The figure shows three views and two pictorial views of one solid part (mm, origin at its lowest corner). Answer the questions. A direction names the side the tool comes from. Coordinates: 2 decimals unless noted, no trailing zeros. Loops run counter-clockwise (first coordinate to the right, second up) from the corner with the lowest first, then second, coordinate; pieces in that order, holes last. Notation, with made-up numbers: (78, 22.5) -> (110, 22.5) arc R33 ccw to (110, 54.5) -> close; hole circle Ø10 at (43.25, -18.75). An arc over 180 degrees is marked (long way). Answer as a JSON object with one key per item and string values. Group by question number.
1) Consider probe 1 along X at (y, z) = (17.5, 16); probe 2 along Y at (x, z) = (56, 30). Determine where each line is inside the solid, lowest interval first. Write a range as [from, to].
2) Section C-C, the plane y = 18.75 is taken. Give the vertices of the cut face in (x, z).
3) Section B-B, the plane z = 30 is taken. Give the vertices of the cut face in (x, y).
4) Which of the six approach directions +Z, -Z, +X, -X, +Y, -Y give full straight-line access (tool end or side, diameter ignored) to the marked faces 1 and 2?
5) Section D-D, the plane z = 44.5 is taken. Give the vertices of the cut face in (x, y), plus the area to 3 significant figures.
6) Section A-A, the plane y = 12.5 is taken. Give the vertices of the cut face in (x, z).
7) Flat-ended cylindrical pins translate along their axes: P1, Ø4, axis at y = 12.5, z = 30, coming from the +X side; P2, Ø1.5, axis at x = 13, z = 33, coming from the +Y side. Find the tip coordinate at first contact, or state that the pin passes through.
8) Determine the mould class of the marked faces 3, 4, 5 and 6 for opening direction Z: released by +Z, released by -Z, zero draft, split by the parting line, or undercut.
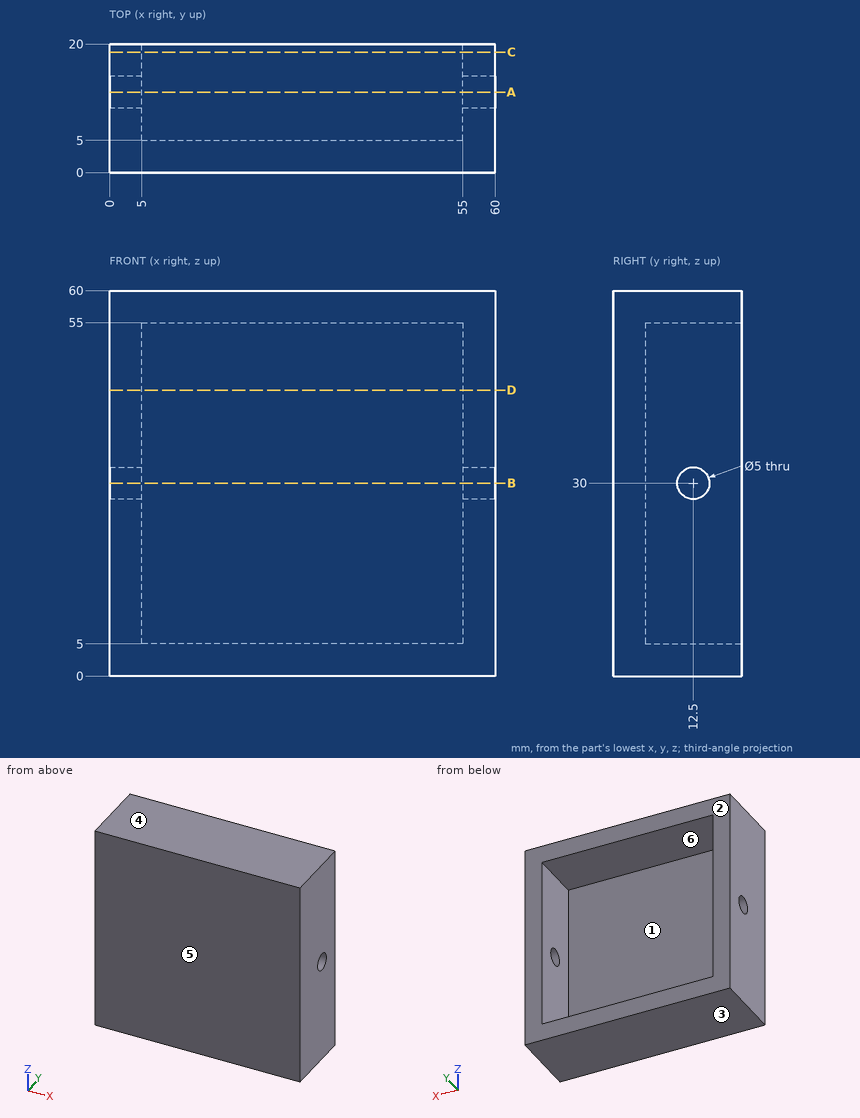
Determined:
{
 "1": {"probe 1": "[0, 5], [55, 60]", "probe 2": "[0, 10], [15, 20]"},
 "2": {"outline": "(0, 0) -> (60, 0) -> (60, 60) -> (0, 60) -> close; hole (5, 5) -> (55, 5) -> (55, 55) -> (5, 55) -> close"},
 "3": {"outline": "(0, 0) -> (60, 0) -> (60, 10) -> (55, 10) -> (55, 5) -> (5, 5) -> (5, 10) -> (0, 10) -> close; (0, 15) -> (5, 15) -> (5, 20) -> (0, 20) -> close; (55, 15) -> (60, 15) -> (60, 20) -> (55, 20) -> close"},
 "4": {"face 1": "+Y", "face 2": "+Z, -Z, +X, -X, +Y"},
 "5": {"outline": "(0, 0) -> (60, 0) -> (60, 20) -> (55, 20) -> (55, 5) -> (5, 5) -> (5, 20) -> (0, 20) -> close", "area": "450 mm²"},
 "6": {"outline": "(0, 0) -> (60, 0) -> (60, 27.5) -> (55, 27.5) -> (55, 5) -> (5, 5) -> (5, 27.5) -> (0, 27.5) -> close; (0, 32.5) -> (5, 32.5) -> (5, 55) -> (55, 55) -> (55, 32.5) -> (60, 32.5) -> (60, 60) -> (0, 60) -> close"},
 "7": {"P1": "through", "P2": "y = 5"},
 "8": {"face 3": "released by -Z", "face 4": "released by +Z", "face 5": "zero draft", "face 6": "undercut"}
}
